Can you work these out from the model? Positions are in its coordinate system, mm. A direction names the side the tool comes from. Round coordinates to 2 decimals unless told otherwise and drop trailing zeros. Loops run counter-clockwise (first coordinate to the right, second up) from the corner with the lowest first, then second, coordinate; pieces in that order, holes last. Notation, with made-up numbers: (74, 19.25) -> (130, 19.25) arc R26 cw to (130, 54.25) -> close; hole circle Ø8 at (-17, 88). An arc over 180 degrees is marked (long way). Write item = value, one per line.
from build123d import *

# Parameters (mm, degrees)
F0_R     = 11
F1_DEPTH = 2
F3_R     = 4.075
F3_R_2   = 2.075
F4_DEPTH = 6
F5_R     = 1.99999
F6_R     = 2


# Not quite as in the source:
# - a fillet or chamfer is up to 0.001 mm smaller than in the source, because OpenCascade refuses the exact size
# - a feature names something its author has since deleted; it is built from what else it names


with BuildPart() as f1:
    # F0 (on Top) → F1 (new body)
    with BuildSketch(Plane.XY):
        with Locations((0, 21.965100023)):
            Circle(F0_R)
    extrude(amount=F1_DEPTH)

    # F3 (on face) → F4 (join)
    with BuildSketch(Plane.XY.offset(2)):
        with Locations((0, 21.965100023)):
            Circle(F3_R)
        with Locations((0, 21.965100023)):
            Circle(F3_R_2, mode=Mode.SUBTRACT)
    extrude(amount=F4_DEPTH)

    # F5 (radius 2 in the source; OpenCascade refuses exactly that, so slightly less here)
    f5_edges = [f1.edges().sort_by_distance(p)[0] for p in [
        (-11, 21.9651, 0),
    ]]
    fillet(f5_edges, radius=F5_R)

    # F6
    f6_edges = [f1.edges().sort_by_distance(p)[0] for p in [
        (-2.075, 21.9651, 2),
    ]]
    fillet(f6_edges, radius=F6_R)


solid = f1.part
1. Suppose I cut it at A-A, the plane z = 5.25. List the corners of the cut face in (x, y) for me (3 decimals).
Entries:
outline = circle Ø8.15 at (0, 21.965); hole circle Ø4.15 at (0, 21.965)
2. We'd pull the mould along X, two halves only. Please class faces 3 (the cylindrical face through (-0.27, 24.022, 5.972)), 4 (the cylindrical face through (-3, 24.72, 4.96)), 5 (the flat face through (-1, 24, 8)): released by +X, released by -X, zero draft, split by the parting line, or undercut.
Entries:
face_3 = undercut
face_4 = split by the parting line
face_5 = zero draft
3. For faces 1 (the flat face through (0, 17, 2)), 2 (the flat face through (0, 22, 0)), which set-ups out of +Z, -Z, +X, -X, +Y, -Y let a thin tool reach every point of the face, with its end or its side?
Entries:
face_1 = +Z
face_2 = -Z, +X, -X, +Y, -Y
4. I need wall thicknesses on line 1 (Y direction, x = 0, z = 5.8); line 2 (Z direction, x = -6.25, y = 16.5); line 3 (X direction, y = 18.25, z = 7.75). Which ranges of each line are inside material? Lowest first, please. Write a range as [from, to].
Entries:
line_1 = [17.89, 19.89], [24.04, 26.04]
line_2 = [0, 2]
line_3 = [-1.67, 1.67]
5. I'm going to push flat-ended pins straight in: pin 1 (1.5 mm diameter, centred on y = 29, z = 2, fed in from -X); pin 2 (3 mm diameter, centred on y = 15.5, z = 1.5, fed in from -X); pin 3 (1 mm diameter, centred on x = 3.5, z = 6, fed in from -Y). Where does each tip first touch, or does it pass through?
Entries:
pin_1 = -9.03
pin_2 = -9.79
pin_3 = 19.21
